Source: CAD feature listing. Evaluate the final solid. Frame: model axes, mm. Face numbers are marked on the shaded views. Round coordinates to 2 decimals unless told otherwise and drop trailing zeros. Loops run counter-clockwise (first coordinate to the right, second up) from the corner with the lowest first, then second, coordinate; pieces in that order, holes last. Notation, with made-up numbers: (-0.75, 61) - (42.25, 61) arc R13 cw to (42.25, 80) - close; hole circle Ø3 at (72.25, 34.25). An arc over 180 degrees is marked (long way). One line per question, with ' | ' between items. Start each with the question number.
1. Cut plane A-A (x = 0). Return loops of the section in (y, z).
2. Cut plane D-D (y = 5.75). Return loops of the section in (x, z), then the cut area to 3 significant figures.
3. Mould query, pull axis Z, two halves, no side actions, for the marked faces 1 and 2. Classes: pulls with the +Z half, pulls with the -Z half, needs draft (parallel to the pull), parting line crosses it, or undercut.
4. Cut plane C-C (y = -1.25). Return loops of the section in (x, z), then the cut area to 3 significant figures.
5. Pin query (flat end, axial travel): pin 1 (5 mm diameter, centred on y = 5, z = 31.5, fed in from +X); pin 2 (4 mm diameter, centred on x = 32.5, y = -1, fed in from +Z); pin 3 (2 mm diameter, centred on y = 3, z = 7, fed in from +X). Return the tip coordinate at first contact, or that it passes through.
6. Ray query, line 1 (X direction, y = 4.5, z = 15.5); line 2 (X direction, y = 1, z = -1.5); line 3 (Y direction, x = 29, z = -3.5). Return the intervals inside material, ascending.
7. Cut plane B-B (z = 0). Return loops of the section in (x, y), then the cut area to 3 significant figures.
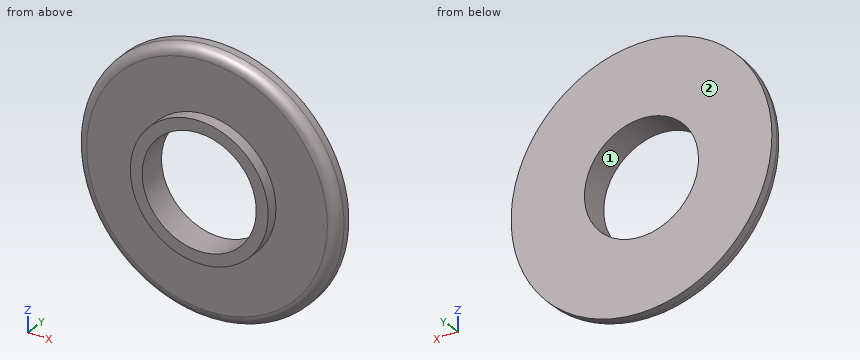
Autodesk Inventor part; units mm, degrees
ref_plane "YZ Plane" through (0, 0, 0) normal (1, 0, 0) x (0, 1, 0)
ref_plane "XZ Plane" through (0, 0, 0) normal (0, 1, 0) x (-1, 0, 0)
ref_plane "XY Plane" through (0, 0, 0) normal (0, 0, 1) x (1, 0, 0)
sketch "Sketch1" plane through (0, 0, 0) normal (0, 1, 0) x (-1, 0, 0)
  circle A0 centre (0, 0) radius 52
  circle A1 centre (0, 0) radius 22.75
  circle A2 centre (0, 0) radius 27.5
  dimension "d2" = 45.5
  dimension "d4" = 55
extrude "Extrusion1" add sketch "Sketch1" against normal blind 4.75 contours A2
extrude "Extrusion2" add sketch "Sketch1" along normal blind 7 contours A0 | A2
fillet "Fillet1" radius 4 1 edges at (52, 0, 0)
properties part number "wheel_chain_guide_holes"
Answers follow:
1) outline: (-4.75, -27.5) - (0, -27.5) - (0, -48) arc R4 ccw to (4, -52) - (7, -52) - (7, -22.75) - (-4.75, -22.75) - close; (-4.75, 22.75) - (7, 22.75) - (7, 52) - (4, 52) arc R4 ccw to (0, 48) - (0, 27.5) - (-4.75, 27.5) - close
2) outline: circle Ø104 at (0, 0); hole circle Ø45.5 at (0, 0) | area: 6,870 mm2
3) face 1: undercut | face 2: needs draft
4) outline: circle Ø55 at (0, 0); hole circle Ø45.5 at (0, 0) | area: 750 mm2
5) pin 1: stops at x = 43.16 | pin 2: stops at z = 39.24 | pin 3: stops at x = 51.61
6) line 1: x = -49.64 to -16.65, 16.65 to 49.64 | line 2: x = -50.62 to -22.7, 22.7 to 50.62 | line 3: y = 0 to 7
7) outline: (-52, 4) arc R4 ccw to (-48, 0) - (-27.5, 0) - (-27.5, -4.75) - (-22.75, -4.75) - (-22.75, 7) - (-52, 7) - close; (22.75, -4.75) - (27.5, -4.75) - (27.5, 0) - (48, 0) arc R4 ccw to (52, 4) - (52, 7) - (22.75, 7) - close | area: 448 mm2
